Here's how the part is built. I have some questions about the finished solid (model axes, mm). A direction names the side the tool comes from. Round coordinates to 2 decimals unless told otherwise and drop trailing zeros. Write each loop counter-clockwise with the first axis right and the second up, starting at its lowest first coordinate (ties: lowest second). Pieces come first, ordered by that corner, then holes. Notation, with made-up numbers: (33.25, 26.5) -> (84.25, 26.5) arc R34 cw to (84.25, 61.5) -> close; hole circle Ø6 at (-26.75, 12). An arc over 180 degrees is marked (long way). Answer in a Markdown table with one row per item. Add a question column.
from build123d import *

# Parameters (mm, degrees)
F1_DEPTH = 304.8
F3_DEPTH = 2540
F4_W     = 762
F4_H     = 304.8
F5_DEPTH = 635


with BuildPart() as f1:
    # F0 (on Top) → F1 (new body)
    with BuildSketch(Plane.XY):
        with BuildLine():
            Line((-1651, 0), (0, 0))
            Line((0, 0), (0, 1270))
            Line((0, 1270), (-1651, 1270))
            Line((-1651, 1270), (-1651, 1268.0179134988))
            ThreePointArc((-1651, 1268.0179134988), (-1203.3887407525, 1082.6112592476), (-1017.9820865012, 635))
            ThreePointArc((-1017.9820865012, 635), (-1203.3887407525, 187.3887407524), (-1651, 1.9820865012))
            Line((-1651, 1.9820865012), (-1651, 0))
        make_face()
        with BuildLine():
            ThreePointArc((-1651, 1268.0179134988), (-2284.0179134988, 635), (-1651, 1.9820865012))
            Line((-1651, 1.9820865012), (-1651, 1268.0179134988))
        make_face()
        with BuildLine():
            Line((-1651, 1268.0179134988), (-1651, 1.9820865012))
            ThreePointArc((-1651, 1.9820865012), (-1203.3887407525, 187.3887407524), (-1017.9820865012, 635))
            ThreePointArc((-1017.9820865012, 635), (-1203.3887407525, 1082.6112592476), (-1651, 1268.0179134988))
        make_face()
    extrude(amount=F1_DEPTH)

    # F2 (on face) → F3 (cut)
    with BuildSketch(Plane.XY.offset(304.8)):
        with BuildLine():
            ThreePointArc((-1333.5, 635), (-1426.4935969733, 859.5064030267), (-1651, 952.5))
            Line((-1651, 952.5), (-1651, 317.5))
            ThreePointArc((-1651, 317.5), (-1426.4935969733, 410.4935969733), (-1333.5, 635))
        make_face()
        with BuildLine():
            Line((-1651, 317.5), (-1651, 952.5))
            ThreePointArc((-1651, 952.5), (-1968.5, 635), (-1651, 317.5))
        make_face()
    extrude(amount=-F3_DEPTH, mode=Mode.SUBTRACT)

    # F4 (on face) → F5 (join)
    with BuildSketch(Plane.XY.offset(304.8)):
        with Locations((-381, 152.4)):
            Rectangle(F4_W, F4_H)
    extrude(amount=F5_DEPTH)


solid = f1.part
Item 1: If we mould it in two halves opening along X, with no side actions, what happens to faces 4 (the flat face through (-654, 0, 359)), 5 (the cylindrical face through (-2283.865, 648.92, 150.266)), 6 (the cylindrical face through (-1865.58, 400.99, 154.53)), 7 (the flat face through (0, 485, 254))? For each: pulls with the +X half, pulls with the -X half, needs draft (parallel to the pull), parting line crosses it, or undercut.
Item 2: If we section it at D-D on x = -228.5: Please give me the cut outline in (y, z), then the cut area to 3 significant figures.
Item 3: I need wall thicknesses on line 1 along X through (y, z) = (635, 172); line 2 along X through (y, z) = (271.5, 586); line 3 along Z through (x, y) = (-786, 1133.5). Which ranges of each line are inside material? Lowest first, please. Write a range as from..to.
Item 4: For P1, Ø2, axis at y = 1269.5, z = 86.5, coming from the -X side; P2, Ø2, axis at y = 232, z = 433, coming from the -X side, each with a flat end and sliding along its axis, tell me the tip position at first contact or that it passes through.
Item 5: If we section it at B-B on x = -1516: Please give me the cut outline in (y, z).
Item 6: If we section it at C-C on z = 784.5: Please give me the cut outline in (x, y).
Item 7: If we section it at A-A on y = 635: Please give me the cut outline in (x, z).
Item 8: On a 3-axis mill with a long thin cutter (end or side, diameter ignored), from which of +Z, -Z, +X, -X, +Y, -Y can I reach the whole of each face in a straight line? I mean faces 1 (the flat face through (-814, 1270, 150)), 2 (the flat face through (-386, 304.8, 618)), 3 (the flat face through (-762, 150, 618)). Say none if no direction works.
Results list:
| question | item | result |
|---|---|---|
| 1 | face 4 | needs draft |
| 1 | face 5 | pulls with the -X half |
| 1 | face 6 | undercut |
| 1 | face 7 | pulls with the +X half |
| 2 | outline | (0, 0) -> (1270, 0) -> (1270, 304.8) -> (304.8, 304.8) -> (304.8, 939.8) -> (0, 939.8) -> close |
| 2 | area | 581,000 mm² |
| 3 | line 1 | -2284.02..-1968.5, -1333.5..0 |
| 3 | line 2 | -762..0 |
| 3 | line 3 | 0..304.8 |
| 4 | P1 | x = -1651 |
| 4 | P2 | x = -762 |
| 5 | outline | (0, 0) -> (347.63, 0) -> (347.63, 304.8) -> (0, 304.8) -> close; (922.37, 0) -> (1270, 0) -> (1270, 304.8) -> (922.37, 304.8) -> close |
| 6 | outline | (-762, 0) -> (0, 0) -> (0, 304.8) -> (-762, 304.8) -> close |
| 7 | outline | (-2284.02, 0) -> (-1968.5, 0) -> (-1968.5, 304.8) -> (-2284.02, 304.8) -> close; (-1333.5, 0) -> (0, 0) -> (0, 304.8) -> (-1333.5, 304.8) -> close |
| 8 | face 1 | +Z, -Z, +X, -X, +Y |
| 8 | face 2 | +Z, +X, -X, +Y |
| 8 | face 3 | +Z, -X, +Y, -Y |
